Can you work these out from the model? Positions are in its coordinate system, mm. Round coordinates to 2 decimals unless told otherwise and drop trailing zeros. Loops run counter-clockwise (first coordinate to the right, second up) from the corner with the lowest first, then second, coordinate; pieces in that order, holes last. Notation, with made-up numbers: M 77,-16 L 99,-16 A20 cw 99,13 Z; hole C 61,63.25 d1. An arc over 180 degrees is marked long. Answer as CSV lines item,"result".
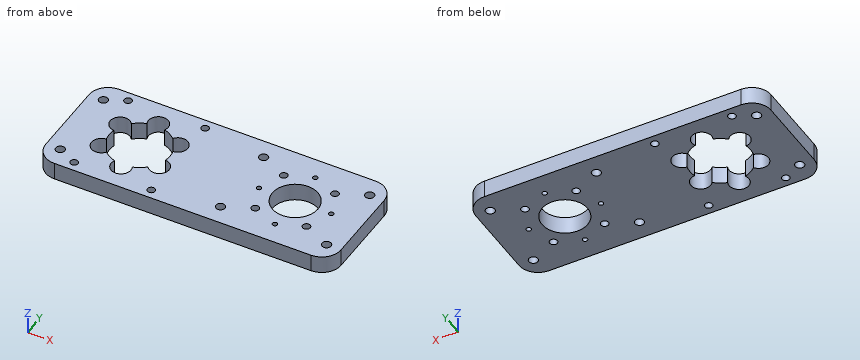
from build123d import *

# Parameters (mm, degrees)
SKETCH1_W                      = 97.2375
SKETCH1_H                      = 38.1
SKETCH1_R                      = 7.5
SKETCH1_R_2                    = 10
BOSS_EXTRUDE1_DEPTH            = 5.8
CBORE_FOR_M3_SHCS1_D           = 3.2
CBORE_FOR_M3_SHCS1_CBORE_D     = 6.5
CBORE_FOR_M3_SHCS1_CBORE_DEPTH = 13
FILLET1_R                      = 6.35
F_4_CLEARANCE_HOLE1_D          = 2.9464
F_4_CLEARANCE_HOLE1_DEPTH      = 5.8
F_4_CLEARANCE_HOLE1_TIP        = 0.885187864
M3X0_5_TAPPED_HOLE1_D          = 2.5
M3X0_5_TAPPED_HOLE1_DEPTH      = 7.5
M3X0_5_TAPPED_HOLE1_TIP        = 0.751075774
M3X0_5_TAPPED_HOLE2_D          = 2.5
M3X0_5_TAPPED_HOLE2_DEPTH      = 8.5
M3X0_5_TAPPED_HOLE2_TIP        = 0.751075774
SKETCH17_R                     = 0.79375
CUT_EXTRUDE3_DEPTH             = 105.596278166


with BuildPart() as part:
    # Sketch1 → Boss-Extrude1 (new body)
    with BuildSketch(Plane.XY):
        with Locations((48.61875, 19.05)):
            Rectangle(SKETCH1_W, SKETCH1_H)
        with Locations((75.0125, 19.05)):
            Circle(SKETCH1_R, mode=Mode.SUBTRACT)
        with Locations((23.8125, 19.05)):
            Circle(SKETCH1_R_2, mode=Mode.SUBTRACT)
    extrude(amount=BOSS_EXTRUDE1_DEPTH)

    # CBORE for M3 SHCS1 (through all)
    with Locations(Plane.XY.offset(5.8)):
        with Locations((33.338779442, 13.55), (33.338779442, 24.55), (23.8125, 30.05), (14.286220558, 24.55), (14.286220558, 13.55), (23.8125, 8.05)):
            CounterBoreHole(CBORE_FOR_M3_SHCS1_D / 2, CBORE_FOR_M3_SHCS1_CBORE_D / 2, CBORE_FOR_M3_SHCS1_CBORE_DEPTH)

    # Fillet1
    fillet1_edges = [part.edges().sort_by_distance(p)[0] for p in [
        (0, 0, 2.9),
        (0, 38.1, 2.9),
        (97.2375, 38.1, 2.9),
        (97.2375, 0, 2.9),
    ]]
    fillet(fillet1_edges, radius=FILLET1_R)

    # #4 Clearance Hole1
    with Locations(Plane.XY.offset(5.8)):
        with Locations((4.7625, 31.75), (4.7625, 6.35), (92.475, 6.35), (92.475, 31.75), (57.55, 31.75), (57.55, 6.35)):
            Hole(F_4_CLEARANCE_HOLE1_D / 2, depth=F_4_CLEARANCE_HOLE1_DEPTH)
            with Locations((0, 0, -(F_4_CLEARANCE_HOLE1_DEPTH + F_4_CLEARANCE_HOLE1_TIP / 2))):  # 118° drill point
                Cone(0, F_4_CLEARANCE_HOLE1_D / 2, F_4_CLEARANCE_HOLE1_TIP, mode=Mode.SUBTRACT)

    # M3x0.5 Tapped Hole1
    with Locations(Plane.XY.offset(5.8)):
        with Locations((11.1125, 34.925), (36.5125, 34.925), (36.5125, 3.175), (11.1125, 3.175)):
            Hole(M3X0_5_TAPPED_HOLE1_D / 2, depth=M3X0_5_TAPPED_HOLE1_DEPTH)
            with Locations((0, 0, -(M3X0_5_TAPPED_HOLE1_DEPTH + M3X0_5_TAPPED_HOLE1_TIP / 2))):  # 118° drill point
                Cone(0, M3X0_5_TAPPED_HOLE1_D / 2, M3X0_5_TAPPED_HOLE1_TIP, mode=Mode.SUBTRACT)

    # M3x0.5 Tapped Hole2
    with Locations(Plane.XY.offset(5.8)):
        with Locations((66.593509886, 27.468990114), (83.431490114, 27.468990114), (83.431490114, 10.631009886), (66.593509886, 10.631009886)):
            Hole(M3X0_5_TAPPED_HOLE2_D / 2, depth=M3X0_5_TAPPED_HOLE2_DEPTH)
            with Locations((0, 0, -(M3X0_5_TAPPED_HOLE2_DEPTH + M3X0_5_TAPPED_HOLE2_TIP / 2))):  # 118° drill point
                Cone(0, M3X0_5_TAPPED_HOLE2_D / 2, M3X0_5_TAPPED_HOLE2_TIP, mode=Mode.SUBTRACT)

    # Sketch17 → Cut-Extrude3 (cut, through all)
    with BuildSketch(Plane.XY.offset(5.8)):
        with Locations((63.10625, 19.05)):
            Circle(SKETCH17_R)
        with Locations((75.0125, 7.14375)):
            Circle(SKETCH17_R)
        with Locations((86.91875, 19.05)):
            Circle(SKETCH17_R)
        with Locations((75.0125, 30.95625)):
            Circle(SKETCH17_R)
    extrude(amount=-CUT_EXTRUDE3_DEPTH, mode=Mode.SUBTRACT)


solid = part.part
Item 1: If we section it at A-A on x = 57.55: Write out the boundary of the cut face in (y, z), then the cut area to 3 significant figures.
Output:
outline,"M 0,0 L 4.88,0 L 4.88,5.8 L 0,5.8 Z; M 7.82,0 L 30.28,0 L 30.28,5.8 L 7.82,5.8 Z; M 33.22,0 L 38.1,0 L 38.1,5.8 L 33.22,5.8 Z"
area,"187 mm2"
Item 2: If we section it at B-B on y = 13.5: Write out the boundary of the cut face in (x, z).
Output:
outline,"M 0,0 L 11.04,0 L 11.04,5.8 L 0,5.8 Z; M 36.59,0 L 69.97,0 L 69.97,5.8 L 36.59,5.8 Z; M 80.06,0 L 97.24,0 L 97.24,5.8 L 80.06,5.8 Z"
Item 3: If I drill on line 1 along X through (y, z) = (27, 3.2); line 2 along X through (y, z) = (30, 3.8); line 3 along Y through (x, z) = (24.5, 5.55), over which ranges is the centre line in solid material (lowest first)? Write a range as from..to.
Output:
line 1,"x = 0..12.15, 16.42..17.75, 29.88..31.2, 35.47..65.43, 67.75..82.27, 84.59..97.24"
line 2,"x = 0..20.56, 27.06..97.24"
line 3,"y = 0..4.87, 33.23..38.1"
Item 4: Will these pins go through, and if not, where does the flat tip stop? pin 1 (2 mm diameter, centred on y = 33, z = 3, fed in from +X); pin 2 (5 mm diameter, centred on x = 33.34, y = 13.55, fed in from +Z).
Output:
pin 1,"stops at x = 97.23"
pin 2,"passes through"
Item 5: If we section it at C-C on x = 16: Write out the boundary of the cut face in (y, z), then the cut area to 3 significant figures.
Output:
outline,"M 0,0 L 10.79,0 L 10.79,5.8 L 0,5.8 Z; M 27.31,0 L 38.1,0 L 38.1,5.8 L 27.31,5.8 Z"
area,"125 mm2"
Item 6: If we section it at D-D on z = 1.15: State how many separate pieces and enclosed holes the cut face has, then the cut area to 3 significant figures.
Output:
separate pieces,"1"
enclosed holes,"20"
area,"2,950 mm2"
